from build123d import *

# Parameters (mm, degrees)
BOSS_EXTRUDE1_DEPTH = 0.9652


with BuildPart() as part:
    # Sketch2 → Boss-Extrude1 (new body)
    with BuildSketch(Plane(origin=(0, 0, 0), x_dir=(1, 0, 0), z_dir=(0, 1, 0))):
        with BuildLine():
            Line((14.732, -0.508), (14.732, 2.54))
            ThreePointArc((14.732, 2.54), (14.620407684, 2.809407684), (14.351, 2.921))
            Line((14.351, 2.921), (6.458532376, 2.921))
            ThreePointArc((6.458532376, 2.921), (6.189124692, 3.032592316), (6.077532376, 3.302))
            Line((6.077532376, 3.302), (6.077532376, 6.495707179))
            Line((6.077532376, 6.495707179), (4.299532376, 6.495707179))
            Line((4.299532376, 6.495707179), (4.299532376, 3.302))
            ThreePointArc((4.299532376, 3.302), (4.187940059, 3.032592316), (3.918532376, 2.921))
            Line((3.918532376, 2.921), (0.5842, 2.921))
            Line((0.5842, 2.921), (-7.0358, 2.921))
            ThreePointArc((-7.0358, 2.921), (-7.647331795, 2.309468205), (-8.258863591, 2.921))
            Line((-8.258863591, 2.921), (-11.594310971, 2.921))
            Line((-11.594310971, 2.921), (-12.723617207, 2.385330376))
            Line((-12.723617207, 2.385330376), (-14.732, 2.385330376))
            Line((-14.732, 2.385330376), (-14.732, -2.385330376))
            Line((-14.732, -2.385330376), (-12.723617207, -2.385330376))
            Line((-12.723617207, -2.385330376), (-11.594310971, -2.921))
            Line((-11.594310971, -2.921), (-8.258863591, -2.921))
            ThreePointArc((-8.258863591, -2.921), (-7.647331795, -2.309468205), (-7.0358, -2.921))
            Line((-7.0358, -2.921), (0.5842, -2.921))
            ThreePointArc((0.5842, -2.921), (0.853607684, -3.032592316), (0.9652, -3.302))
            Line((0.9652, -3.302), (0.9652, -5.207))
            Line((0.9652, -5.207), (3.048, -7.747))
            Line((3.048, -7.747), (4.9022, -5.207))
            Line((4.9022, -5.207), (4.9022, -2.921))
            Line((4.9022, -2.921), (4.9022, -1.27))
            ThreePointArc((4.9022, -1.27), (5.013792316, -1.000592316), (5.2832, -0.889))
            Line((5.2832, -0.889), (14.351, -0.889))
            ThreePointArc((14.351, -0.889), (14.620407684, -0.777407684), (14.732, -0.508))
        make_face()
    extrude(amount=BOSS_EXTRUDE1_DEPTH)


solid = part.part
For this review, take the finished solid that the model builds, in its own axes (mm). A direction names the side the tool comes from. Coordinates: 2 decimals unless noted, no trailing zeros. Loops run counter-clockwise (first coordinate to the right, second up) from the corner with the lowest first, then second, coordinate; pieces in that order, holes last. Notation, with made-up numbers: (-6, 25.25) -> (41, 25.25) arc R18 ccw to (41, 60.25) -> close; hole circle Ø5 at (58.5, 46). An arc over 180 degrees is marked (long way). Write each question's results on one line, items separated by ' | '.
Q1. To check wall thickness, follow line 1 along Z through (x, y) = (12, 0.25); line 2 along X through (y, z) = (0.15, -6); line 3 along Z through (x, y) = (-10.25, 0.15). State the ranges of each line that lie inside material, in increasing order. Write a range as [from, to].
Taken from the geometry:
line 1: [-2.92, 0.89] | line 2: [4.3, 6.08] | line 3: [-2.92, 2.92]
Q2. Mouldability with a two-part tool opening along X and no side actions: class faces 1 (the cylindrical face through (-7.63, 0.48, -2.31)), 2 (the flat face through (3.962, 0.476, 6.495)), 3 (the flat face through (0, 0, 1)) as +X half, -X half, draft (parallel to the pull), parting line (faces both ways), or undercut.
Taken from the geometry:
face 1: undercut | face 2: +X half | face 3: draft
Q3. Add section C-C, the plane x = 12.25. State the section outline as (y, z) points, then the cut area to 3 significant figures.
Taken from the geometry:
outline: (0, -2.92) -> (0.97, -2.92) -> (0.97, 0.89) -> (0, 0.89) -> close | area: 3.68 mm²
Q4. Machinability: for faces 4 (the flat face through (4.3, 0.5, -4.9)), 5 (the flat face through (10.5, 0.5, -2.921)), 6 (the flat face through (4.902, 0.5, 3.3)), 7 (the flat face through (-3.3, 0.5, 2.921)), which of the approach directions +Z, -Z, +X, -X, +Y, -Y give a long, thin tool a straight path to every point of the face, cutting with its end or side? Answer none if there is none.
Taken from the geometry:
face 4: -Z, -X, +Y, -Y | face 5: -Z, +X, +Y, -Y | face 6: +Z, +X, +Y, -Y | face 7: +Z, -X, +Y, -Y
Q5. Add section A-A, the plane y = 0.8. State the section outline as (x, z) points, then the cut area to 3 significant figures.
Taken from the geometry:
outline: (-14.73, -2.39) -> (-12.72, -2.39) -> (-11.59, -2.92) -> (-8.26, -2.92) arc R0.61 cw to (-7.04, -2.92) -> (3.92, -2.92) arc R0.38 cw to (4.3, -3.3) -> (4.3, -6.5) -> (6.08, -6.5) -> (6.08, -3.3) arc R0.38 cw to (6.46, -2.92) -> (14.35, -2.92) arc R0.38 ccw to (14.73, -2.54) -> (14.73, 0.51) arc R0.38 ccw to (14.35, 0.89) -> (5.28, 0.89) arc R0.38 cw to (4.9, 1.27) -> (4.9, 5.21) -> (3.05, 7.75) -> (0.97, 5.21) -> (0.97, 3.3) arc R0.38 cw to (0.58, 2.92) -> (-7.04, 2.92) arc R0.61 cw to (-8.26, 2.92) -> (-11.59, 2.92) -> (-12.72, 2.39) -> (-14.73, 2.39) -> close | area: 169 mm²
Q6. Add section B-B, the plane x = -4. State the section outline as (y, z) points.
Taken from the geometry:
outline: (0, -2.92) -> (0.97, -2.92) -> (0.97, 2.92) -> (0, 2.92) -> close
Q7. For pin 1 Ø0.5 at (x, y) = (-1.5, 0.5) entering from +Z; pin 2 Ø0.5 at (y, z) = (0.5, -4) entering from -X; pin 3 Ø0.5 at (x, y) = (-10, 0.5) entering from -Z, all flat-tipped, find the tip position at first contact; note any pin that passes through.
Taken from the geometry:
pin 1: z = 2.92 | pin 2: x = 4.3 | pin 3: z = -2.92
